Could you check a few things on this model? Use its own coordinates, in mm. Face numbers are marked on the shaded views. A direction names the side the tool comes from. Coordinates: 2 decimals unless noted, no trailing zeros. Write each loop counter-clockwise with the first axis right and the second up, starting at its lowest first coordinate (ties: lowest second). Pieces come first, ordered by that corner, then holes.
Item 1: I want a section at D-D on x = -4.8. Please give me the cut outline in (y, z) (3 decimals).
Item 2: Which directions (+Z, -Z, +X, -X, +Y, -Y) give clear straight access to the entire face, cutting with the end or side of a thin tool? Please do the marked faces 4, 5, 6 and 7.
Item 3: Thinking about a two-plate mould opening in Y: for the marked faces 1, 2 and 3, which applies, +Y half, -Y half, draft (parallel to the pull), parting line (faces both ways), or undercut?
Item 4: I want a section at B-B on x = 1.5. Please give me the cut outline in (y, z).
Item 5: If I drill on probe 1 along X at (y, z) = (-1, 2.2) (3 decimals); probe 2 along Y at (x, z) = (9, -10); probe 3 along Z at (x, y) = (7.25, 1.5), over which ranges is the centre line in solid material (lowest first)?
Item 6: I want a section at C-C on z = 2.2. Please give me the cut outline in (x, y) (3 decimals).
Item 7: I want a section at A-A on y = 0. State how many separate pieces and enclosed holes the cut face has, then the cut area to 3 significant figures.
Item 8: For P1, Ø2.5, axis at y = 0.5, z = 7, coming from the -X side; P2, Ø2.5, axis at y = 1, z = -9, coming from the +X side; P3, Ø1.4, axis at x = 4.7, z = 2.2, coming from the +Y side; P4, Ø1, axis at y = 0.5, z = 6.5, coming from the +X side, each with a flat end and sliding along its axis, tell me the tip position at first contact or that it passes through.
from build123d import *

# Parameters (mm, degrees)
EXTRUDE_1_DEPTH     = 3.2
CUT_EXTRUDE_1_REACH = 14.844
SKETCH_2_R          = 1.175
FILLET_1_R          = 0.5
EXTRUDE_1_2_DEPTH   = 2.5
EXTRUDE_2_DEPTH     = 0.3
EXTRUDE_3_REACH     = 19.807
SKETCH_5_R          = 0.6
SKETCH_6_R          = 2.4
EXTRUDE_4_DEPTH     = 1.6
CHAMFER_1_SIZE      = 0.2
SKETCH_7_W          = 0.2
SKETCH_7_H          = 3.5
EXTRUDE_2_2_DEPTH   = 1.6


with BuildPart() as part:
    # 草图1 → Extrude 1 (new, symmetric)
    with BuildSketch(Plane(origin=(0, 0, 0), x_dir=(1, 0, 0), z_dir=(0, 1, 0))):
        Polygon((9.9, 4.4), (0, 4.4), (-0.7, 5.1), (-9.9, 5.1), (-9.9, -5.1), (9.9, -5.1), align=None)
    extrude(amount=EXTRUDE_1_DEPTH, both=True)

    # 草图2 → 切除-拉伸1 (cut, up to next)
    with BuildSketch(Plane(origin=(0, 3.2, 0), x_dir=(1, 0, 0), z_dir=(0, 1, 0)), mode=Mode.PRIVATE) as cut_extrude_1_sk1:
        with Locations(Location((-4.8, -2.2, 0), (0, 0, 270))):
            Circle(SKETCH_2_R)
    cut_extrude_1_tool1 = extrude(cut_extrude_1_sk1.sketch, amount=-CUT_EXTRUDE_1_REACH, mode=Mode.PRIVATE) & part.part
    # 草图2 → 切除-拉伸1 (cut, up to next)
    with BuildSketch(Plane(origin=(0, 3.2, 0), x_dir=(1, 0, 0), z_dir=(0, 1, 0)), mode=Mode.PRIVATE) as cut_extrude_1_sk2:
        with Locations(Location((4.7, -2.2, 0), (0, 0, 270))):
            Circle(SKETCH_2_R)
    cut_extrude_1_tool2 = extrude(cut_extrude_1_sk2.sketch, amount=-CUT_EXTRUDE_1_REACH, mode=Mode.PRIVATE) & part.part
    add(cut_extrude_1_tool1.solids().sort_by_distance((-4.8, 3.2, 2.2))[0], mode=Mode.SUBTRACT)
    add(cut_extrude_1_tool2.solids().sort_by_distance((4.7, 3.2, 2.2))[0], mode=Mode.SUBTRACT)

    # 圆角1
    fillet_1_edges = [part.edges().sort_by_distance(p)[0] for p in [
        (9.9, 0, 5.1),
        (-9.9, 0, 5.1),
        (-9.9, 0, -5.1),
        (9.9, 0, -4.4),
    ]]
    fillet(fillet_1_edges, radius=FILLET_1_R)

    # 草图3 → Extrude 1 2 (add, symmetric)
    with BuildSketch(Plane(origin=(0, 0, 0), x_dir=(1, 0, 0), z_dir=(0, 1, 0))):
        with BuildLine():
            Line((-6.75, 5.1), (-6.75, 5.85))
            ThreePointArc((-6.75, 5.85), (-6.574264069, 6.274264069), (-6.15, 6.45))
            Line((-6.15, 6.45), (11.7, 6.45))
            Line((11.7, 6.45), (11.7, 6.75))
            Line((11.7, 6.75), (-6.15, 6.75))
            ThreePointArc((-6.15, 6.75), (-6.786396103, 6.486396103), (-7.05, 5.85))
            Line((-7.05, 5.85), (-7.05, 5.1))
            Line((-7.05, 5.1), (-6.75, 5.1))
        make_face()
    extrude(amount=EXTRUDE_1_2_DEPTH, both=True)

    # 草图4 → Extrude 2 (add)
    with BuildSketch(Plane(origin=(0, 2.5, 0), x_dir=(1, 0, 0), z_dir=(0, 1, 0))):
        with BuildLine():
            Line((7.7, 9.8), (7.7, 6.45))
            Line((7.7, 6.45), (11.7, 6.45))
            Line((11.7, 6.45), (11.7, 9.8))
            ThreePointArc((11.7, 9.8), (9.7, 11.8), (7.7, 9.8))
        make_face()
    extrude_2 = extrude(amount=-EXTRUDE_2_DEPTH)

    # 镜向1: Extrude 2 across plane
    add(extrude_2.mirror(Plane.ZX))

    # 凸台-拉伸3: up to this face of the body (flat: up to its plane)
    extrude_3_end = Plane(part.part.faces().sort_by_distance((-0.181890176, -3.2, 0.080625265))[0])
    # 草图5 → 凸台-拉伸3 (add, up to the picked face)
    with BuildSketch(Plane(origin=(0, 3.2, 0), x_dir=(1, 0, 0), z_dir=(0, 1, 0)), mode=Mode.PRIVATE) as extrude_3_sk1:
        with Locations(Location((9.7, 9.8, 0), (0, 0, 270))):
            Circle(SKETCH_5_R)
    extrude_3_tool1 = split(extrude(extrude_3_sk1.sketch, amount=-EXTRUDE_3_REACH, mode=Mode.PRIVATE), bisect_by=extrude_3_end, keep=Keep.BOTH, mode=Mode.PRIVATE)
    add(extrude_3_tool1.solids().sort_by(Axis((9.7, 3.2, -9.8), (0, -1, 0)))[0])

    # 草图6 → 凸台-拉伸4 (add, symmetric)
    with BuildSketch(Plane(origin=(0, 0, 0), x_dir=(1, 0, 0), z_dir=(0, 1, 0))):
        with Locations(Location((9.7, 9.8, 0), (0, 0, 270))):
            Circle(SKETCH_6_R)
    extrude(amount=EXTRUDE_4_DEPTH, both=True)

    # 倒角1
    chamfer_1_edges = [part.edges().sort_by_distance(p)[0] for p in [
        (9.7, -1.6, -12.2),
        (9.7, 1.6, -12.2),
    ]]
    chamfer(chamfer_1_edges, length=CHAMFER_1_SIZE)

    # 草图7 → Extrude 2 2 (add, symmetric)
    with BuildSketch(Plane(origin=(0, 0, 0), x_dir=(1, 0, 0), z_dir=(0, 1, 0))):
        with Locations((-8.2, -6.85)):
            Rectangle(SKETCH_7_W, SKETCH_7_H)
        with Locations((0.6, -6.85)):
            Rectangle(SKETCH_7_W, SKETCH_7_H)
        with Locations((7.9, -6.85)):
            Rectangle(SKETCH_7_W, SKETCH_7_H)
    extrude(amount=EXTRUDE_2_2_DEPTH, both=True)


solid = part.part
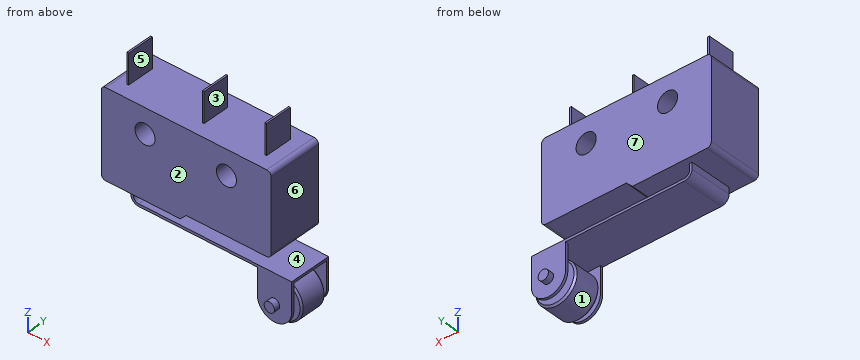
Response values:
1. outline: (-3.2, -5.1) - (3.2, -5.1) - (3.2, 1.025) - (-3.2, 1.025) - close; (-3.2, 3.375) - (3.2, 3.375) - (3.2, 5.1) - (-3.2, 5.1) - close; (-2.5, -6.75) - (2.5, -6.75) - (2.5, -6.45) - (-2.5, -6.45) - close
2. face 4: +X, +Y, -Y
2. face 5: +Z, +Y, -Y
2. face 6: +Z, +X, +Y, -Y
2. face 7: +Z, -Z, +X, -X, +Y
3. face 1: undercut
3. face 2: -Y half
3. face 3: draft
4. outline: (-3.2, -4.4) - (3.2, -4.4) - (3.2, 5.1) - (-3.2, 5.1) - close; (-2.5, -6.75) - (2.5, -6.75) - (2.5, -6.45) - (-2.5, -6.45) - close
5. probe 1: x = -9.9 to -5.975, -3.625 to 3.525, 5.875 to 9.9
5. probe 2: y = -2.5 to -2.2, -1.6 to 1.6, 2.2 to 2.5
5. probe 3: z = -6.75 to -6.45, -4.4 to 5.1
6. outline: (-9.9, -3.2) - (-5.975, -3.2) - (-5.975, 3.2) - (-9.9, 3.2) - close; (-3.625, -3.2) - (3.525, -3.2) - (3.525, 3.2) - (-3.625, 3.2) - close; (5.875, -3.2) - (9.9, -3.2) - (9.9, 3.2) - (5.875, 3.2) - close
7. separate pieces: 2
7. enclosed holes: 2
7. area: 212 mm2
8. P1: stops at x = -8.3
8. P2: stops at x = 12.1
8. P3: passes through
8. P4: stops at x = 8
